Check sheet for the modelled part. Datum: model origin and axes. Units: mm. A direction names the side the tool comes from. Give positions to 0.01 mm unless a question says otherwise; leave off trailing zeros. Order: outer loops, then holes, each group sorted by start corner. A loop starts at its lowest first (then second) coordinate and runs counter-clockwise, first axis right, second up.
```python
from build123d import *

# Parameters (mm, degrees)
BOSS_EXTRU_1_DEPTH      = 3
CONG_1_R                = 5
ESQUISSE2_R             = 1
ESQUISSE2_R_2           = 1.5
ENL_V_MAT_EXTRU_1_DEPTH = 257.837010573
D_GAGEMENT_M31_D        = 3.4
ESQUISSE5_W             = 45
ESQUISSE5_H             = 25
ESQUISSE5_W_2           = 33
ESQUISSE5_H_2           = 90
ESQUISSE5_W_3           = 22
ESQUISSE5_H_3           = 55
ESQUISSE5_W_4           = 30
ESQUISSE5_H_4           = 60
ESQUISSE5_W_5           = 20
ESQUISSE5_H_5           = 47.5
ENL_V_MAT_EXTRU_2_DEPTH = 257.837010573
CONG_2_R                = 3


with BuildPart() as part:
    # Esquisse1 → Boss.-Extru.1 (new body)
    with BuildSketch(Plane(origin=(0, 0, 0), x_dir=(1, 0, 0), z_dir=(0, 1, 0))):
        Polygon((-92.5, 0), (92.5, 0), (132.5, 40), (132.5, 220), (102.5, 220), (85.179491924, 190), (-85.179491924, 190), (-102.5, 220), (-132.5, 220), (-132.5, 40), align=None)
    extrude(amount=BOSS_EXTRU_1_DEPTH)

    # Congé1
    cong_1_edges = [part.edges().sort_by_distance(p)[0] for p in [
        (92.5, 1.5, 0),
        (-92.5, 1.5, 0),
        (-132.5, 1.5, -40),
        (-132.5, 1.5, -220),
        (-102.5, 1.5, -220),
        (-85.179491924, 1.5, -190),
        (85.179491924, 1.5, -190),
        (102.5, 1.5, -220),
        (132.5, 1.5, -220),
        (132.5, 1.5, -40),
    ]]
    fillet(cong_1_edges, radius=CONG_1_R)

    # Esquisse2 → Enlèv. mat.-Extru.1 (cut, through all)
    with BuildSketch(Plane.XZ):
        with Locations(Location((-70, -8, 0), (0, 0, 270))):
            Circle(ESQUISSE2_R)
        with Locations(Location((-124.5, -70, 0), (0, 0, 270))):
            Circle(ESQUISSE2_R)
        with Locations(Location((-124.5, -212, 0), (0, 0, 270))):
            Circle(ESQUISSE2_R)
        with Locations(Location((124.5, -212, 0), (0, 0, 90))):
            Circle(ESQUISSE2_R)
        with Locations(Location((124.5, -70, 0), (0, 0, 90))):
            Circle(ESQUISSE2_R)
        with Locations(Location((70, -8, 0), (0, 0, 90))):
            Circle(ESQUISSE2_R)
        with Locations(Location((126, -50, 0), (0, 0, 270))):
            Circle(ESQUISSE2_R_2)
        with Locations(Location((126, -200, 0), (0, 0, 270))):
            Circle(ESQUISSE2_R_2)
        with Locations(Location((-60, -6.5, 0), (0, 0, 270))):
            Circle(ESQUISSE2_R_2)
        with Locations(Location((60, -6.5, 0), (0, 0, 270))):
            Circle(ESQUISSE2_R_2)
        with Locations(Location((-126, -50, 0), (0, 0, 270))):
            Circle(ESQUISSE2_R_2)
        with Locations(Location((-126, -200, 0), (0, 0, 270))):
            Circle(ESQUISSE2_R_2)
        with Locations(Location((-119.5, -185, 0), (0, 0, 270))):
            Circle(ESQUISSE2_R_2)
        with Locations(Location((-22.5, -185, 0), (0, 0, 270))):
            Circle(ESQUISSE2_R_2)
        with Locations(Location((-101, -72, 0), (0, 0, 270))):
            Circle(ESQUISSE2_R_2)
        with Locations(Location((-37.5, -72, 0), (0, 0, 270))):
            Circle(ESQUISSE2_R_2)
    extrude(amount=-ENL_V_MAT_EXTRU_1_DEPTH, mode=Mode.SUBTRACT)

    # Dégagement M31 (through all)
    with Locations(Plane(origin=(0, 0, 0), x_dir=(-1, 0, 0), z_dir=(0, -1, 0))):
        with Locations((-70, 8), (-124.5, 70), (-124.5, 212), (124.5, 212), (124.5, 70), (70, 8), (-126, 200), (-126, 50), (-60, 6.5), (60, 6.5), (126, 50), (126, 200), (101, 72), (37.5, 72), (119.5, 185), (22.5, 185)):
            Hole(D_GAGEMENT_M31_D / 2)

    # Esquisse5 → Enlèv. mat.-Extru.2 (cut, through all)
    with BuildSketch(Plane.XZ):
        with Locations((45, -177.5)):
            Rectangle(ESQUISSE5_W, ESQUISSE5_H)
        with Locations((-9, -127)):
            Rectangle(ESQUISSE5_W_2, ESQUISSE5_H_2)
        with Locations((95.5, -52.5)):
            Rectangle(ESQUISSE5_W_3, ESQUISSE5_H_3)
        with Locations((35.5, -54)):
            Rectangle(ESQUISSE5_W_4, ESQUISSE5_H_4)
        with Locations((-67.5, -38.75)):
            Rectangle(ESQUISSE5_W_5, ESQUISSE5_H_5)
        with Locations((97.5, -121.25)):
            Rectangle(ESQUISSE5_W_4, ESQUISSE5_H_5)
    extrude(amount=-ENL_V_MAT_EXTRU_2_DEPTH, mode=Mode.SUBTRACT)

    # Congé2
    cong_2_edges = [part.edges().sort_by_distance(p)[0] for p in [
        (-77.5, 1.5, -62.5),
        (-77.5, 1.5, -15),
        (-57.5, 1.5, -15),
        (-57.5, 1.5, -62.5),
        (84.5, 1.5, -80),
        (84.5, 1.5, -25),
        (106.5, 1.5, -25),
        (106.5, 1.5, -80),
        (20.5, 1.5, -84),
        (20.5, 1.5, -24),
        (50.5, 1.5, -24),
        (50.5, 1.5, -84),
        (-25.5, 1.5, -172),
        (-25.5, 1.5, -82),
        (7.5, 1.5, -82),
        (7.5, 1.5, -172),
        (82.5, 1.5, -145),
        (82.5, 1.5, -97.5),
        (112.5, 1.5, -97.5),
        (112.5, 1.5, -145),
        (22.5, 1.5, -190),
        (22.5, 1.5, -165),
        (67.5, 1.5, -165),
        (67.5, 1.5, -190),
    ]]
    fillet(cong_2_edges, radius=CONG_2_R)


solid = part.part
```
(1) Release check for a two-part mould opening along X. For faces 3 (the face through (-93.739, 1.479, -204.825)), 4 (the face through (-112.8, 1.5, -20.3)), 5 (the face through (-31, 0, -112)) record: released by +X, released by -X, zero draft, split by the parting line, or undercut.
Response values:
face 3: undercut
face 4: released by -X
face 5: zero draft
(2) Set-up check for faces 1 (the face through (93.941, 1.479, -205.175)), 2 (the face through (112.2, 1.5, -19.7)): record each of +Z, -Z, +X, -X, +Y, -Y from which the full face is reachable in a straight line by a thin tool's end or side.
Response values:
face 1: -Z, +Y, -Y
face 2: +Z, +X, +Y, -Y
(3) Gauge pin test, flat ends, axial feed: pin 1 Ø1.5 at (x, y) = (49, 1) entering from -Z; pin 2 Ø0.9 at (x, y) = (93, 2) entering from -Z; pin 3 Ø1.5 at (x, y) = (-54.5, 1.5) entering from -Z. Record the tip position at first contact, or that the pin passes through.
Response values:
pin 1: stops at z = -165
pin 2: stops at z = -204.32
pin 3: stops at z = -190
(4) Material ranges on L1, parallel to X at y = 1.85, z = -70; L2, parallel to X at y = 0.4, z = -44; L3, parallel to X at y = 0.7, z = -74, recorded low to high.
Response values:
L1: x = -132.5 to -126.2, -122.8 to 20.5, 50.5 to 84.5, 106.5 to 122.8, 126.2 to 132.5
L2: x = -132.5 to -77.5, -57.5 to 20.5, 50.5 to 84.5, 106.5 to 132.5
L3: x = -132.5 to 20.5, 50.5 to 84.5, 106.5 to 132.5
(5) Cross-section at B-B on x = 29. Enter the section's corners in (y, z).
Response values:
outline: (0, -165) - (3, -165) - (3, -84) - (0, -84) - close; (0, -24) - (3, -24) - (3, 0) - (0, 0) - close
(6) Cross-section at C-C on y = 1.65. Count the separate pieces of the cut face and the enclosed holes in it, then the cut area to 3 significant figures.
Response values:
separate pieces: 1
enclosed holes: 21
area: 41,500 mm2
(7) Cross-section at A-A on z = -129.5. Enter the section's corners in (x, y).
Response values:
outline: (-132.5, 0) - (-25.5, 0) - (-25.5, 3) - (-132.5, 3) - close; (7.5, 0) - (82.5, 0) - (82.5, 3) - (7.5, 3) - close; (112.5, 0) - (132.5, 0) - (132.5, 3) - (112.5, 3) - close
